Could you check a few things on this model? Use its own coordinates, in mm. A direction names the side the tool comes from. Give positions to 0.01 mm unless a question says otherwise; leave off trailing zeros. Order: outer loops, then holes, each group sorted by start corner. A loop starts at its lowest first (then second) coordinate and runs counter-clockwise, first axis right, second up. Notation, with made-up numbers: (9.5, 74.25) -> (40.5, 74.25) arc R27 cw to (40.5, 105.25) -> close; hole circle Ø5 at (7.25, -33). An arc over 180 degrees is marked (long way). Answer as CSV lines item,"result". Start each with the question number.
(1) I want a section at B-B (x = 0). Please give me the cut outline in (y, z) (3 decimals).
(2) I want a section at A-A (z = 6.25). Please give me the cut outline in (x, y) (3 decimals), plus the area to 3 significant figures.
(3) On a 3-axis mill with a long thin cutter (end or side, diameter ignored), from which of +Z, -Z, +X, -X, +Y, -Y can I reach the whole of each face in a straight line? I mean faces 1 (the face through (-1.02, -3.6, 3.7)), 2 (the face through (30, 0, 3)). Say none if no direction works.
(4) Will these pins go through, and if not, where does the flat tip stop? pin 1 Ø8 at (x, y) = (14, -4) entering from -Z; pin 2 Ø1 at (y, z) = (-4.5, 6) entering from -X; pin 3 Ø0.6 at (x, z) = (0.5, 4.5) entering from -Y.
(5) I want a section at C-C (y = 0). Please give me the cut outline in (x, z) (3 decimals).
(6) I need wall thicknesses on L1, parallel to Y at x = 0, z = 9.2 (3 decimals); L2, parallel to Y at x = 0, z = 3 (3 decimals); L3, parallel to Z at x = 26, y = -4.25. Which ranges of each line are inside material? Lowest first, please.
(7) I want a section at D-D (z = 4.25). Please give me the cut outline in (x, y) (3 decimals).
(8) We'd pull the mould along X, two halves only. Please class faces 3 (the face through (3.6, -1.02, 3.7)), 4 (the face through (13.835, -6.241, 2.972)), 5 (the face through (-1.427, -6.428, 7.465)), 6 (the face through (-4, 0, 0)): released by +X, released by -X, zero draft, split by the parting line, or undercut.
```python
from build123d import *

# Parameters (mm, degrees)
BOSS_EXTRUDE3_DEPTH = 5
SKETCH3_R           = 6.585
BOSS_EXTRUDE4_DEPTH = 5
SKETCH5_R           = 4.185
CUT_EXTRUDE1_DEPTH  = 7.5
SKETCH4_W           = 2.04
SKETCH4_H           = 1.02
SKETCH4_W_2         = 1.02
SKETCH4_H_2         = 2.04
BOSS_EXTRUDE5_DEPTH = 7.5
SKETCH6_R           = 1.36
CUT_EXTRUDE2_DEPTH  = 2.5
SKETCH7_R           = 6.585
CUT_EXTRUDE3_DEPTH  = 1
FILLET1_R           = 0.5


with BuildPart() as part:
    # Sketch1 → Boss-Extrude3 (new body)
    with BuildSketch(Plane.XY):
        with BuildLine():
            Line((1.173518627, 8.08022766), (26.146764706, 4.453279176))
            ThreePointArc((26.146764706, 4.453279176), (30, 0), (26.146764706, -4.453279176))
            Line((26.146764706, -4.453279176), (1.173518627, -8.08022766))
            ThreePointArc((1.173518627, -8.08022766), (-8.165, 0), (1.173518627, 8.08022766))
        make_face()
    extrude(amount=BOSS_EXTRUDE3_DEPTH)

    # Sketch3 → Boss-Extrude4 (add)
    with BuildSketch(Plane.XY.offset(5)):
        Circle(SKETCH3_R)
    extrude(amount=BOSS_EXTRUDE4_DEPTH)

    # Sketch5 → Cut-Extrude1 (cut)
    with BuildSketch(Plane(origin=(0, 0, 0), x_dir=(-1, 0, 0), z_dir=(0, 0, -1))):
        Circle(SKETCH5_R)
    extrude(amount=-CUT_EXTRUDE1_DEPTH, mode=Mode.SUBTRACT)

    # Sketch4 → Boss-Extrude5 (add)
    with BuildSketch(Plane(origin=(0, 0, 0), x_dir=(-1, 0, 0), z_dir=(0, 0, -1))):
        with Locations((0, 3.675)):
            Rectangle(SKETCH4_W, SKETCH4_H)
        with Locations((3.675, 0)):
            Rectangle(SKETCH4_W_2, SKETCH4_H_2)
        with Locations((0, -3.675)):
            Rectangle(SKETCH4_W, SKETCH4_H)
        with Locations((-3.675, 0)):
            Rectangle(SKETCH4_W_2, SKETCH4_H_2)
    extrude(amount=-BOSS_EXTRUDE5_DEPTH)

    # Sketch6 → Cut-Extrude2 (cut)
    with BuildSketch(Plane.XY.offset(10)):
        Circle(SKETCH6_R)
    extrude(amount=-CUT_EXTRUDE2_DEPTH, mode=Mode.SUBTRACT)

    # Sketch7 → Cut-Extrude3 (cut)
    with BuildSketch(Plane(origin=(0, 0, 0), x_dir=(-1, 0, 0), z_dir=(0, 0, -1))):
        with BuildLine():
            Line((-26.146764706, 4.453279176), (-1.173518627, 8.08022766))
            ThreePointArc((-1.173518627, 8.08022766), (8.165, 0), (-1.173518627, -8.08022766))
            Line((-1.173518627, -8.08022766), (-26.146764706, -4.453279176))
            ThreePointArc((-26.146764706, -4.453279176), (-30, 0), (-26.146764706, 4.453279176))
        make_face()
        with Locations(Location((0, 0, 0), (0, 0, 180))):
            Circle(SKETCH7_R, mode=Mode.SUBTRACT)
    extrude(amount=-CUT_EXTRUDE3_DEPTH, mode=Mode.SUBTRACT)

    # Fillet1
    fillet1_edges = [part.edges().sort_by_distance(p)[0] for p in [
        (-6.585, 0, 0),
    ]]
    fillet(fillet1_edges, radius=FILLET1_R)


solid = part.part
```
Final values:
1,outline,"(-8.165, 1) -> (-6.585, 1) -> (-6.585, 0.5) arc R0.5 ccw to (-6.085, 0) -> (-3.165, 0) -> (-3.165, 7.5) -> (-1.36, 7.5) -> (-1.36, 10) -> (-6.585, 10) -> (-6.585, 5) -> (-8.165, 5) -> close; (1.36, 7.5) -> (3.165, 7.5) -> (3.165, 0) -> (6.085, 0) arc R0.5 ccw to (6.585, 0.5) -> (6.585, 1) -> (8.165, 1) -> (8.165, 5) -> (6.585, 5) -> (6.585, 10) -> (1.36, 10) -> close"
2,outline,"circle Ø13.17 at (0, 0); hole (-4.059, -1.02) arc R4.185 ccw to (-1.02, -4.059) -> (-1.02, -3.165) -> (1.02, -3.165) -> (1.02, -4.059) arc R4.185 ccw to (4.059, -1.02) -> (3.165, -1.02) -> (3.165, 1.02) -> (4.059, 1.02) arc R4.185 ccw to (1.02, 4.059) -> (1.02, 3.165) -> (-1.02, 3.165) -> (-1.02, 4.059) arc R4.185 ccw to (-4.059, 1.02) -> (-3.165, 1.02) -> (-3.165, -1.02) -> close"
2,area,"89.2 mm²"
3,face 1,"-Z"
3,face 2,"+Z, -Z, +X"
4,pin 1,"z = 1"
4,pin 2,"x = -5.23"
4,pin 3,"y = -8.16"
5,outline,"(-8.165, 1) -> (-6.585, 1) -> (-6.585, 0.5) arc R0.5 ccw to (-6.085, 0) -> (-3.165, 0) -> (-3.165, 7.5) -> (-1.36, 7.5) -> (-1.36, 10) -> (-6.585, 10) -> (-6.585, 5) -> (-8.165, 5) -> close; (1.36, 7.5) -> (3.165, 7.5) -> (3.165, 0) -> (6.085, 0) arc R0.5 ccw to (6.585, 0.5) -> (6.585, 1) -> (30, 1) -> (30, 5) -> (6.585, 5) -> (6.585, 10) -> (1.36, 10) -> close"
6,L1,"-6.585 to -1.36, 1.36 to 6.585"
6,L2,"-8.165 to -3.165, 3.165 to 8.165"
6,L3,"1 to 5"
7,outline,"(1.174, -8.08) -> (26.147, -4.453) arc R4.5 ccw to (26.147, 4.453) -> (1.174, 8.08) arc R8.165 ccw (long way) to start; hole (-4.059, -1.02) arc R4.185 ccw to (-1.02, -4.059) -> (-1.02, -3.165) -> (1.02, -3.165) -> (1.02, -4.059) arc R4.185 ccw to (4.059, -1.02) -> (3.165, -1.02) -> (3.165, 1.02) -> (4.059, 1.02) arc R4.185 ccw to (1.02, 4.059) -> (1.02, 3.165) -> (-1.02, 3.165) -> (-1.02, 4.059) arc R4.185 ccw to (-4.059, 1.02) -> (-3.165, 1.02) -> (-3.165, -1.02) -> close"
8,face 3,"undercut"
8,face 4,"released by +X"
8,face 5,"split by the parting line"
8,face 6,"zero draft"
